Input: part model. Units: mm. Frame: model coordinates. A direction names the side the tool comes from. Coordinates: 2 decimals unless noted, no trailing zeros. Order: outer loops, then holes, each group sorted by start corner. A loop starts at its lowest first (then second) coordinate and runs counter-clockwise, first axis right, second up. Notation, with made-up numbers: (41.5, -27) -> (73.5, -27) arc R14 ccw to (73.5, -10) -> close; hole circle Ø6 at (57.25, 31). An arc over 180 degrees is marked (long way). One line per question, with ' | ' between items.
```python
from build123d import *

# Parameters (mm, degrees)
SKETCH1_W           = 200
SKETCH1_H           = 200
BOSS_EXTRUDE1_DEPTH = 10
SKETCH2_W           = 120
SKETCH2_H           = 120
SKETCH2_W_2         = 100
SKETCH2_H_2         = 100
CUT_EXTRUDE1_DEPTH  = 1
FILLET1_R           = 5


with BuildPart() as part:
    # Sketch1 → Boss-Extrude1 (new body)
    with BuildSketch(Plane(origin=(0, 0, 0), x_dir=(1, 0, 0), z_dir=(0, 1, 0))):
        Rectangle(SKETCH1_W, SKETCH1_H)
    extrude(amount=BOSS_EXTRUDE1_DEPTH)

    # Sketch2 → Cut-Extrude1 (cut)
    with BuildSketch(Plane(origin=(0, 10, 0), x_dir=(1, 0, 0), z_dir=(0, 1, 0))):
        Rectangle(SKETCH2_W, SKETCH2_H)
        Rectangle(SKETCH2_W_2, SKETCH2_H_2, mode=Mode.SUBTRACT)
        with BuildLine():
            Line((-35, 5), (35, 5))
            ThreePointArc((35, 5), (40, 0), (35, -5))
            Line((35, -5), (20, -5))
            Line((20, -5), (20, -35))
            ThreePointArc((20, -35), (15, -40), (10, -35))
            Line((10, -35), (10, -5))
            Line((10, -5), (-10, -5))
            Line((-10, -5), (-10, -35))
            ThreePointArc((-10, -35), (-15, -40), (-20, -35))
            Line((-20, -35), (-20, -5))
            Line((-20, -5), (-35, -5))
            ThreePointArc((-35, -5), (-40, 0), (-35, 5))
        make_face()
    extrude(amount=-CUT_EXTRUDE1_DEPTH, mode=Mode.SUBTRACT)

    # Fillet1
    fillet1_edges = [part.edges().sort_by_distance(p)[0] for p in [
        (20, 9.5, 5),
        (10, 9.5, 5),
        (-10, 9.5, 5),
        (-20, 9.5, 5),
        (-60, 9.5, 60),
        (-60, 9.5, -60),
        (60, 9.5, -60),
        (60, 9.5, 60),
    ]]
    fillet(fillet1_edges, radius=FILLET1_R)


solid = part.part
```
1. Access query for faces 5 (the face through (-1, 0, -1)), 6 (the face through (-58.5, 9.49, 58.57)). Directions: +Z, -Z, +X, -X, +Y, -Y. A direction counts if a zero-diameter tool reaches every point of the face in a straight line with its end or side. Return the directions, or none.
Recorded:
face 5: +Z, -Z, +X, -X, -Y | face 6: +Y
2. Pin query (flat end, axial travel): pin 1 Ø8 at (x, z) = (-49, -12) entering from -Y. Return the tip coordinate at first contact, or that it passes through.
Recorded:
pin 1: stops at y = 0
3. Cut plane B-B, the plane z = 0. Return loops of the section in (x, y), and give its area (3 significant figures).
Recorded:
outline: (-100, 0) -> (100, 0) -> (100, 10) -> (60, 10) -> (60, 9) -> (50, 9) -> (50, 10) -> (40, 10) -> (40, 9) -> (-40, 9) -> (-40, 10) -> (-50, 10) -> (-50, 9) -> (-60, 9) -> (-60, 10) -> (-100, 10) -> close | area: 1,900 mm^2
4. Cut plane A-A, the plane x = 15. Return loops of the section in (y, z).
Recorded:
outline: (0, -100) -> (10, -100) -> (10, -60) -> (9, -60) -> (9, -50) -> (10, -50) -> (10, -5) -> (9, -5) -> (9, 40) -> (10, 40) -> (10, 50) -> (9, 50) -> (9, 60) -> (10, 60) -> (10, 100) -> (0, 100) -> close
5. Cut plane C-C, the plane z = 23.5. Return loops of the section in (x, y), and give its area (3 significant figures).
Recorded:
outline: (-100, 0) -> (100, 0) -> (100, 10) -> (60, 10) -> (60, 9) -> (50, 9) -> (50, 10) -> (20, 10) -> (20, 9) -> (10, 9) -> (10, 10) -> (-10, 10) -> (-10, 9) -> (-20, 9) -> (-20, 10) -> (-50, 10) -> (-50, 9) -> (-60, 9) -> (-60, 10) -> (-100, 10) -> close | area: 1,960 mm^2
6. Ray query, line 1 (Z direction, x = -25, y = 9.25); line 2 (Y direction, x = 23.5, z = -4). Return the intervals inside material, ascending. Write a range as [from, to].
Recorded:
line 1: z = [-100, -60], [-50, -5], [5, 50], [60, 100] | line 2: y = [0, 9]
7. Mould query, pull axis Z, two halves, no side actions, for faces 1 (the face through (-100, 5, 1)), 2 (the face through (1, 9, 2)), 3 (the face through (-1, 5, 100)), 4 (the face through (40, 9.5, -0.1)). Classes: released by +Z, released by -Z, zero draft, split by the parting line, or undercut.
Recorded:
face 1: zero draft | face 2: undercut | face 3: released by +Z | face 4: undercut
